from build123d import *

# Parameters (mm, degrees)
F1_DEPTH = 63.5
F2_DEPTH = 25.4
F0_W     = 23.1578589316
F0_H     = 19.05
F3_DEPTH = 25.4
F4_DEPTH = 7.9375
F6_R     = 6.35


with BuildPart() as f1:
    # F0 (on Front) → F1 (new body, symmetric)
    with BuildSketch(Plane.XZ):
        Polygon((-41.275, 9.525), (-41.275, -9.525), (41.275, -9.525), (41.275, 9.525), (22.225, 9.525), align=None)
    extrude(amount=F1_DEPTH, both=True)

    # F0 (on Front) → F2 (join, symmetric)
    with BuildSketch(Plane.XZ):
        with BuildLine():
            Line((22.225, 9.525), (41.275, 9.525))
            Line((41.275, 9.525), (41.275, 27.0002))
            ThreePointArc((41.275, 27.0002), (45.9246798487, 38.2255201513), (57.15, 42.8752))
            Line((57.15, 42.8752), (60.325, 42.8752))
            Line((60.325, 42.8752), (60.325, 61.9252))
            Line((60.325, 61.9252), (57.15, 61.9252))
            ThreePointArc((57.15, 61.9252), (32.4542956671, 51.6959043329), (22.225, 27.0002))
            Line((22.225, 27.0002), (22.225, 9.525))
        make_face()
    extrude(amount=F2_DEPTH, both=True)

    # F0 (on Front) → F3 (join, symmetric)
    with BuildSketch(Plane.XZ):
        with Locations((71.9039294658, 52.4002)):
            Rectangle(F0_W, F0_H)
    extrude(amount=F3_DEPTH, both=True)

    # F0 (on Front) → F4 (join, symmetric)
    with BuildSketch(Plane.XZ):
        with BuildLine():
            add(Edge.make_bspline(
                [(-41.275, 9.525), (-41.1813110113, 44.7291582823), (16.6801214218, 63.2801502943), (57.15, 61.9252)],
                knots=[0, 0, 0, 0, 111.5045361635, 111.5045361635, 111.5045361635, 111.5045361635], degree=3))
            Line((-41.275, 9.525), (22.225, 9.525))
            Line((22.225, 9.525), (22.225, 27.0002))
            ThreePointArc((22.225, 27.0002), (32.4542956671, 51.6959043329), (57.15, 61.9252))
        make_face()
    extrude(amount=F4_DEPTH, both=True)

    # F0 (on Front) → F5 (revolve)
    with BuildSketch(Plane.XZ):
        Polygon((83.4828589316, 66.675), (83.4828589316, 61.9252), (83.4828589316, 42.8752), (83.4828589316, 38.1), (111.125, 38.1), (111.125, 66.675), align=None)
    revolve(axis=Axis((83.4828589316, 0, 52.3875), (0, 0, -1)))

    # F6
    f6_edges = [f1.edges().sort_by_distance(p)[0] for p in [
        (-41.275, -63.5, 0),
        (41.275, -63.5, 0),
        (41.275, 63.5, 0),
        (-41.275, 63.5, 0),
    ]]
    fillet(f6_edges, radius=F6_R)


solid = f1.part
Model file for the job. Use its own axes, mm. A direction names the side the tool comes from. Give positions to 0.01 mm unless a question says otherwise; leave off trailing zeros. Loops run counter-clockwise (first coordinate to the right, second up) from the corner with the lowest first, then second, coordinate; pieces in that order, holes last. Notation, with made-up numbers: (-18.5, 56) - (2.5, 56) arc R14 ccw to (2.5, 78) - close; hole circle Ø10 at (37, 21). An arc over 180 degrees is marked (long way). Use one line per item in the form item = value.
(1) Cut at A-A (z = -4.5). Give the cut face in (x, y) (3 decimals).
Determined:
outline = (-41.275, -57.15) arc R6.35 ccw to (-34.925, -63.5) - (34.925, -63.5) arc R6.35 ccw to (41.275, -57.15) - (41.275, 57.15) arc R6.35 ccw to (34.925, 63.5) - (-34.925, 63.5) arc R6.35 ccw to (-41.275, 57.15) - close
(2) Drill centre lines: L1, parallel to X at y = -41.5, z = 8 (3 decimals); L2, parallel to Z at x = 10, y = 39 (3 decimals); L3, parallel to Y at x = 41, z = 26.5. Where is each one in solid material? Low to high.
Determined:
L1 = -41.275 to 41.275
L2 = -9.525 to 9.525
L3 = -25.4 to 25.4
(3) Cut at C-C (x = 80). Give the cut face in (y, z) (3 decimals), then the cut area to 3 significant figures.
Determined:
outline = (-27.422, 38.1) - (27.422, 38.1) - (27.422, 66.675) - (-27.422, 66.675) - close
area = 1,570 mm^2
(4) Cut at D-D (y = 18). Give the cut face in (x, z) (3 decimals), then the cut area to 3 significant figures.
Determined:
outline = (-41.275, -9.525) - (41.275, -9.525) - (41.275, 27) arc R15.875 cw to (57.15, 42.875) - (62.505, 42.875) - (62.505, 38.1) - (104.461, 38.1) - (104.461, 66.675) - (62.505, 66.675) - (62.505, 61.925) - (57.15, 61.925) arc R34.925 ccw to (22.225, 27) - (22.225, 9.525) - (-41.275, 9.525) - close
area = 3,970 mm^2
(5) 3-axis set-ups, long thin cutter, end or side, ignore diameter. For faces 1 (the face through (61, 21, 61.925)), 2 (the face through (84, 0, 38.1)), 3 (the face through (83, 0, 66.675)), 4 (the face through (61, -21, 42.875)), 5 (the face through (61, -21, 61.925)): which of +Z, -Z, +X, -X, +Y, -Y reach the whole face in a straight line?
Determined:
face_1 = +Z, -X, +Y
face_2 = -Z, +X, +Y, -Y
face_3 = +Z, +X, -X, +Y, -Y
face_4 = -Z, -Y
face_5 = +Z, -X, -Y
(6) Drop flat-ended pins along their axis: P1, Ø12.5, axis at x = 61.5, y = 13, coming from the -Z side; P2, Ø12, axis at x = -24.5, z = 49.5, coming from the +Y side; P3, Ø15.5, axis at x = -14, z = 33.5, coming from the +Y side; P4, Ø8, axis at x = 19, z = 16.5, coming from the -Y side. Give the stop position or say it passes through.
Determined:
P1 = 38.1
P2 = through
P3 = 7.94
P4 = -25.4
(7) Cut at B-B (y = -11). Give the cut face in (x, z) (3 decimals), then the cut area to 3 significant figures.
Determined:
outline = (-41.275, -9.525) - (41.275, -9.525) - (41.275, 27) arc R15.875 cw to (57.15, 42.875) - (58.124, 42.875) - (58.124, 38.1) - (108.842, 38.1) - (108.842, 66.675) - (58.124, 66.675) - (58.124, 61.925) - (57.15, 61.925) arc R34.925 ccw to (22.225, 27) - (22.225, 9.525) - (-41.275, 9.525) - close
area = 4,130 mm^2
(8) Pull direction X, two halves, no side cores. Call faces 6 (the face through (32.73, -16.79, 51.97)), 7 (the face through (61, 21, 42.875)), 8 (the face through (-2, -7.938, 31)), 9 (the face through (45.8, -0.4, 38.1)): pulls with the +X half, pulls with the -X half, needs draft (parallel to the pull), parting line crosses it, or undercut.
Determined:
face_6 = pulls with the -X half
face_7 = undercut
face_8 = needs draft
face_9 = undercut
